from build123d import *

# Parameters (mm, degrees)
F1_DEPTH = 7.112


# Not quite as in the source:
# - ends of sketch curves that miss each other by under 0.0002 mm in the source are joined
# - a feature names something its author has since deleted; it is built from what else it names


with BuildPart() as f1:
    # F0 (on Top) → F1 (new body)
    with BuildSketch(Plane.XY):
        with BuildLine():
            ThreePointArc((0, 11.1125), (7.8577241059, 7.8577241059), (11.1125, 0))
            ThreePointArc((11.1125, 0), (10.7338507446, -2.8761266387), (9.6237072996, -5.55625))
            Line((9.6237072996, -5.55625), (12.0983748909, -6.985))
            ThreePointArc((12.0983748909, -6.985), (13.4939838315, -3.6157019175), (13.97, 0))
            ThreePointArc((13.97, 0), (13.4755323786, 3.6838739276), (12.0271328398, 7.1069666985))
            ThreePointArc((12.0271328398, 7.1069666985), (6.9237480813, 12.133532565), (-1.95e-08, 13.97))
            Line((-1.95e-08, 13.97), (0, 11.1125))
        make_face()
        with BuildLine():
            ThreePointArc((-9.6237072996, -5.55625), (-9.6237072996, 5.55625), (0, 11.1125))
            Line((0, 11.1125), (0, 13.97))
            ThreePointArc((-1.95e-08, 13.97), (-6.9237478038, 12.1335327234), (-12.0271324949, 7.1069672823))
            ThreePointArc((-12.0271324949, 7.1069672823), (-13.9698214779, 0.0706248839), (-12.0983748909, -6.985))
            Line((-12.0983748909, -6.985), (-9.6237072996, -5.55625))
        make_face()
        with BuildLine():
            Line((12.0983748909, -6.985), (9.6237072996, -5.55625))
            ThreePointArc((9.6237072996, -5.55625), (0, -11.1125), (-9.6237072996, -5.55625))
            Line((-9.6237072996, -5.55625), (-12.0983748909, -6.985))
            ThreePointArc((-12.0983748909, -6.985), (-7.0460734842, -12.0629079602), (-0.1412475033, -13.969285921))
            ThreePointArc((-0.1412475033, -13.969285921), (6.9237481232, -12.1335325411), (12.0983748909, -6.985))
        make_face()
        with BuildLine():
            ThreePointArc((-8.6769039474, 16.9913819188), (-4.593947408, 14.7469507993), (-1.95e-08, 13.97))
            Line((0, 13.97), (0, 16.8275))
            ThreePointArc((0, 16.8275), (-3.65427634, 17.4455290423), (-6.9020826854, 19.2308719809))
            Line((-6.9020826854, 19.2308719809), (-8.6769039474, 16.9913819188))
        make_face()
        with BuildLine():
            ThreePointArc((-12.0271324949, 7.1069672823), (-6.9237478038, 12.1335327234), (-1.95e-08, 13.97))
            ThreePointArc((-1.95e-08, 13.97), (-4.593947408, 14.7469507993), (-8.6769039474, 16.9913819188))
            ThreePointArc((-8.6769039474, 16.9913819188), (-9.8388621787, 11.8752452293), (-12.0271324949, 7.1069672823))
        make_face()
        with BuildLine():
            Line((0, 16.8275), (0, 13.97))
            ThreePointArc((-1.95e-08, 13.97), (4.5939473896, 14.7469507929), (8.6769039474, 16.9913819188))
            ThreePointArc((8.6769039474, 16.9913819188), (12.5773059147, 21.8595168015), (13.97, 27.94))
            Line((13.97, 27.94), (11.1125, 27.94))
            ThreePointArc((11.1125, 27.94), (7.8577241059, 20.0822758941), (0, 16.8275))
        make_face()
        with BuildLine():
            ThreePointArc((19.4187283795, -0.8424940876), (15.2170069875, -3.2683590347), (12.0983750385, -6.9849997443))
            Line((12.0983750385, -6.9849997443), (14.5730424822, -8.41375))
            ThreePointArc((14.5730424822, -8.41375), (21.320623143, -3.2361492554), (29.7529997817, -4.3462927004))
            Line((29.7529997817, -4.3462927004), (31.1817497817, -1.8716251091))
            ThreePointArc((31.1817497817, -1.8716251091), (25.4143155079, -0.0531600677), (19.4187283795, -0.8424940876))
        make_face()
        with BuildLine():
            ThreePointArc((13.97, 0), (13.4939838315, -3.6157019175), (12.0983750385, -6.9849997443))
            ThreePointArc((12.0983750385, -6.9849997443), (15.2170069875, -3.2683590347), (19.4187283795, -0.8424940876))
            ThreePointArc((19.4187283795, -0.8424940876), (15.2933094518, 2.7327644521), (12.0271328398, 7.1069666985))
            ThreePointArc((12.0271328398, 7.1069666985), (13.4755323786, 3.6838739276), (13.97, 0))
        make_face()
        with BuildLine():
            Line((14.5730424822, -8.41375), (12.0983748909, -6.985))
            ThreePointArc((12.0983748909, -6.985), (10.4389854978, -11.5441348126), (10.4389854722, -16.395865042))
            ThreePointArc((10.4389854722, -16.395865042), (12.753195723, -21.9828628158), (17.2117497817, -26.0683748909))
            Line((17.2117497817, -26.0683748909), (18.6404997817, -23.5937072996))
            ThreePointArc((18.6404997817, -23.5937072996), (13.4628990371, -16.8461266387), (14.5730424822, -8.41375))
        make_face()
        with BuildLine():
            ThreePointArc((-10.2267497817, -13.97), (-10.7027659885, -10.3542979399), (-12.0983748909, -6.985))
            Line((-12.0983748909, -6.985), (-14.5730424822, -8.41375))
            ThreePointArc((-14.5730424822, -8.41375), (-13.4628990371, -11.0938733613), (-13.0842497817, -13.97))
            ThreePointArc((-13.0842497817, -13.97), (-14.5730424822, -19.52625), (-18.6404997817, -23.5937072996))
            Line((-18.6404997817, -23.5937072996), (-17.2117497817, -26.0683748909))
            ThreePointArc((-17.2117497817, -26.0683748909), (-12.6422439072, -21.8220248341), (-10.3765164134, -16.010110204))
            ThreePointArc((-10.3765164134, -16.010110204), (-10.2642417492, -14.9928000402), (-10.2267497817, -13.97))
        make_face()
        with BuildLine():
            ThreePointArc((-0.1412475033, -13.969285921), (-7.0460734842, -12.0629079602), (-12.0983748909, -6.985))
            ThreePointArc((-12.0983748909, -6.985), (-10.7027659885, -10.3542979399), (-10.2267497817, -13.97))
            ThreePointArc((-10.2267497817, -13.97), (-10.2642417492, -14.9928000402), (-10.3765164134, -16.010110204))
            ThreePointArc((-10.3765164134, -16.010110204), (-5.36483273, -14.4583271608), (-0.1412475033, -13.969285921))
        make_face()
        with BuildLine():
            Line((-14.5730424822, -8.41375), (-12.0983748909, -6.985))
            ThreePointArc((-12.0983748909, -6.985), (-15.2170068744, -3.2683591296), (-19.4187283795, -0.8424940876))
            Line((-19.4187283795, -0.8424940876), (-20.396050939, -3.5276657515))
            ThreePointArc((-20.396050939, -3.5276657515), (-17.0537724691, -5.4573311258), (-14.5730424822, -8.41375))
        make_face()
        with BuildLine():
            ThreePointArc((8.6769039474, 16.9913819188), (9.8388622875, 11.8752449082), (12.0271328398, 7.1069666985))
            ThreePointArc((12.0271328398, 7.1069666985), (15.2933094518, 2.7327644521), (19.4187283795, -0.8424940876))
            Line((19.4187283795, -0.8424940876), (13.97, 27.94))
            ThreePointArc((13.97, 27.94), (12.5773059147, 21.8595168015), (8.6769039474, 16.9913819188))
        make_face()
        with BuildLine():
            ThreePointArc((-19.4187283795, -0.8424940876), (-15.293309221, 2.7327647003), (-12.0271324949, 7.1069672823))
            ThreePointArc((-12.0271324949, 7.1069672823), (-9.8388621787, 11.8752452293), (-8.6769039474, 16.9913819188))
            Line((-8.6769039474, 16.9913819188), (-31.1817497817, -1.8716251091))
            ThreePointArc((-31.1817497817, -1.8716251091), (-27.8124518418, -0.4760162067), (-24.1967497817, 0))
            ThreePointArc((-24.1967497817, 0), (-21.7708847397, -0.2122356904), (-19.4187283795, -0.8424940876))
        make_face()
        with BuildLine():
            ThreePointArc((-13.97, 27.94), (-12.5773059147, 21.8595168015), (-8.6769039474, 16.9913819188))
            Line((-8.6769039474, 16.9913819188), (-6.9020826854, 19.2308719809))
            ThreePointArc((-6.9020826854, 19.2308719809), (-10.0046751594, 23.1032520012), (-11.1125, 27.94))
            Line((-11.1125, 27.94), (-13.97, 27.94))
        make_face()
        with BuildLine():
            ThreePointArc((10.4389854722, -16.395865042), (5.2800111814, -14.6107766948), (-0.1412475033, -13.969285921))
            ThreePointArc((-0.1412475033, -13.969285921), (-5.36483273, -14.4583271608), (-10.3765164134, -16.010110204))
            Line((-10.3765164134, -16.010110204), (17.2117497817, -26.0683748909))
            ThreePointArc((17.2117497817, -26.0683748909), (12.753195723, -21.9828628158), (10.4389854722, -16.395865042))
        make_face()
        with BuildLine():
            Line((-20.396050939, -3.5276657515), (-19.4187283795, -0.8424940876))
            ThreePointArc((-19.4187283795, -0.8424940876), (-21.7708847397, -0.2122356904), (-24.1967497817, 0))
            Line((-24.1967497817, 0), (-24.1967497817, -2.8575))
            ThreePointArc((-24.1967497817, -2.8575), (-22.2670844074, -3.0263238447), (-20.396050939, -3.5276657515))
        make_face()
        with BuildLine():
            ThreePointArc((-11.1125, 27.94), (0, 39.0525), (11.1125, 27.94))
            Line((11.1125, 27.94), (13.97, 27.94))
            ThreePointArc((13.97, 27.94), (0, 41.91), (-13.97, 27.94))
            Line((-13.97, 27.94), (-11.1125, 27.94))
        make_face()
        with BuildLine():
            Line((-29.7529997817, -4.3462927004), (-31.1817497817, -1.8716251091))
            ThreePointArc((-31.1817497817, -1.8716251091), (-36.2951246726, -20.955), (-17.2117497817, -26.0683748909))
            Line((-17.2117497817, -26.0683748909), (-18.6404997817, -23.5937072996))
            ThreePointArc((-18.6404997817, -23.5937072996), (-33.8204570813, -19.52625), (-29.7529997817, -4.3462927004))
        make_face()
        with BuildLine():
            ThreePointArc((-24.1967497817, 0), (-27.8124518418, -0.4760162067), (-31.1817497817, -1.8716251091))
            Line((-31.1817497817, -1.8716251091), (-29.7529997817, -4.3462927004))
            ThreePointArc((-29.7529997817, -4.3462927004), (-27.0728764204, -3.2361492554), (-24.1967497817, -2.8575))
            Line((-24.1967497817, -2.8575), (-24.1967497817, 0))
        make_face()
        with BuildLine():
            Line((31.1817497817, -1.8716251091), (29.7529997817, -4.3462927004))
            ThreePointArc((29.7529997817, -4.3462927004), (33.8204570813, -8.41375), (35.3092497817, -13.97))
            ThreePointArc((35.3092497817, -13.97), (29.7529997817, -23.5937072996), (18.6404997817, -23.5937072996))
            Line((18.6404997817, -23.5937072996), (17.2117497817, -26.0683748909))
            ThreePointArc((17.2117497817, -26.0683748909), (31.1817497817, -26.0683748909), (38.1667497817, -13.97))
            ThreePointArc((38.1667497817, -13.97), (36.2951246726, -6.985), (31.1817497817, -1.8716251091))
        make_face()
    extrude(amount=F1_DEPTH)


solid = f1.part
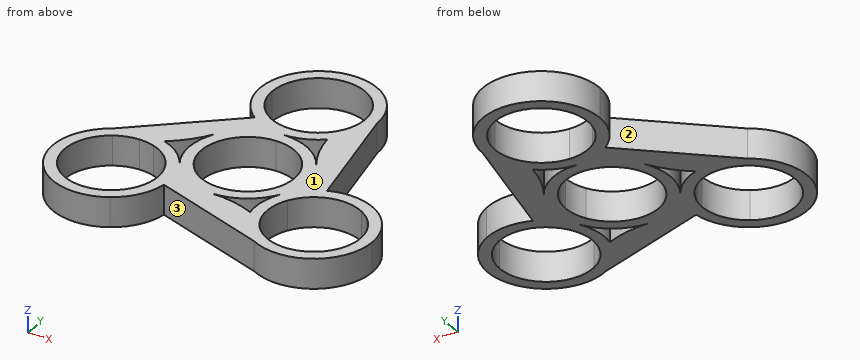
The listing builds one solid part. Answer for the finished solid, in the listing's coordinates (mm). Face numbers are marked on the shaded views. Round coordinates to 2 decimals unless told otherwise and drop trailing zeros. Write each loop counter-clockwise with the first axis right and the second up, starting at its lowest first coordinate (ties: lowest second). Pieces come first, ordered by that corner, then holes. Notation, with made-up numbers: M 1.25,-26 L 45.25,-26 A32 ccw 45.25,5 Z; hole C -39,87.5 d5. An arc over 180 degrees is marked long. Write each question's results on one line, items separated by ' | '. Start each with the question number.
Item 1: Straight lines are drawn through the part: L1, parallel to X at y = 28.5, z = 4.25; L2, parallel to X at y = -2.5, z = 3.75; L3, parallel to Y at x = -17, z = 4. For each, find the intervals that lie inside material, in ascending order. Write a range as [from, to].
Item 2: A cutting plane is placed at D-D on z = 6.25. Write down the section's boundary in (x, y) (1 decimal), and give its area (3 significant figures).
Item 3: A cutting plane is placed at B-B on x = 27.5. Write down the section's boundary in (y, z).
Item 4: A cutting plane is placed at C-C on x = 3. Write down the section's boundary in (y, z), and give its area (3 significant figures).
Item 5: For a pull along X with two mould halves and no side action, classify the marked faces 1, 2 and 3 as pulls with the +X half, pulls with the -X half, needs draft (parallel to the pull), parting line crosses it, or undercut.
Item 6: Flat-ended cylindrical pins translate along their axes: pin 1 Ø12 at (x, y) = (22.5, 24) entering from -Z; pin 2 Ø1 at (x, z) = (-12, 1) entering from +Y. Find the tip coordinate at first contact, or state that the pin passes through.
Item 7: A cutting plane is placed at A-A on y = 29.5. Write down the section's boundary in (x, z).
Check sheet entries:
1) L1: [-13.96, -11.1], [11.1, 13.96] | L2: [-32.17, -16.22], [-13.74, -10.83], [10.83, 32.17] | L3: [-25.94, -22.44], [-5.5, -2], [1.06, 10.02]
2) outline: M -31.2,-1.9 A14 ccw long -10.4,-16 L 17.2,-26.1 A14 ccw long 19.4,-0.8 L 14,27.9 A14 ccw long -8.7,17 Z; hole C -24.2,-14 d22.2; hole M -19.4,-0.8 A14 cw -12.1,-7 A14 cw -12,7.1 A25.4 cw Z; hole C 0,0 d22.2; hole C 0,27.9 d22.2; hole M -0.1,-14 A25.4 cw 10.4,-16.4 A14 cw 12.1,-7 A14 cw Z; hole M 0,14 A14 cw 12,7.1 A25.4 cw 8.7,17 A14 cw Z; hole C 24.2,-14 d22.2 | area: 1,340 mm²
3) outline: M -27.54,0 L -24.58,0 L -24.58,7.11 L -27.54,7.11 Z; M -3.36,0 L -0.4,0 L -0.4,7.11 L -3.36,7.11 Z
4) outline: M -20.89,0 L -14.2,0 L -14.2,7.11 L -20.89,7.11 Z; M -13.64,0 L -10.7,0 L -10.7,7.11 L -13.64,7.11 Z; M 10.7,0 L 13.64,0 L 13.64,7.11 L 10.7,7.11 Z; M 14.3,0 L 17.24,0 L 17.24,7.11 L 14.3,7.11 Z; M 38.64,0 L 41.58,0 L 41.58,7.11 L 38.64,7.11 Z | area: 131 mm²
5) face 1: needs draft | face 2: pulls with the -X half | face 3: undercut
6) pin 1: through | pin 2: y = 35.87
7) outline: M -13.88,0 L -11,0 L -11,7.11 L -13.88,7.11 Z; M 11,0 L 13.88,0 L 13.88,7.11 L 11,7.11 Z
